Model file for the job. Use its own axes, mm. Face numbers are marked on the shaded views. A direction names the side the tool comes from. Round coordinates to 2 decimals unless told otherwise and drop trailing zeros. Loops run counter-clockwise (first coordinate to the right, second up) from the corner with the lowest first, then second, coordinate; pieces in that order, holes last. Notation, with made-up numbers: M -31.75,65.5 L 8.25,65.5 A21 ccw 8.25,85.5 Z; hole C 6,-9.75 d3. An arc over 180 degrees is marked long. Use a Markdown table: item, result. Add a question column.
Q1. Cut at B-B (x = 114.3). Give the cut face in (y, z), plus the area to 3 significant figures.
Q2. Mould opens along Y. For the marked faces 3, 4 and 5 say: +Y half, -Y half, draft (parallel to the pull), parting line (faces both ways), or undercut.
Q3. Cut at C-C (x = 76.5). Give the cut face in (y, z), plus the area to 3 significant figures.
Q4. Cut at A-A (z = 6.5). Give the cut face in (x, y).
Q5. Tool access for the marked faces 1 and 2: list every direction of +Z, -Z, +X, -X, +Y, -Y with a clear straight run to the whole face (end or side of a thin tool).
Q6. Cut at D-D (x = 57.5). Give the cut face in (y, z), plus the area to 3 significant figures.
Q7. Probe line 1 (Y direction, x = 60, z = 12.5); line 2 (Y direction, x = 99, z = 11.25); line 3 (Z direction, x = 114, y = 1). List the from-to ranges inside material, lowest first. Write a range as from..to.
Q8. Pin check, flat tips, straight feed: pin 1 (1 mm diameter, centred on x = 85.5, y = 18.5, fed in from +Z); pin 2 (7 mm diameter, centred on y = 92.5, z = 16, fed in from +X); pin 3 (2 mm diameter, centred on x = 69.5, z = 12, fed in from -Y); pin 4 (3 mm diameter, centred on x = 49.5, y = 143, fed in from +Z). Stop position of each tip, or through.
from build123d import *

# Parameters (mm, degrees)
SKETCH1_W           = 127
SKETCH1_H           = 147.574
BOSS_EXTRUDE1_DEPTH = 3.81
SKETCH3_W           = 127
SKETCH3_H           = 6.35
BOSS_EXTRUDE2_DEPTH = 16.51
SKETCH4_R           = 3.429
CUT_EXTRUDE1_DEPTH  = 196.754917885
SKETCH6_W           = 12.7
SKETCH6_H           = 6.35
BOSS_EXTRUDE3_DEPTH = 18.796
CUT_EXTRUDE4_DEPTH  = 6.35


with BuildPart() as part:
    # Sketch1 → Boss-Extrude1 (new body)
    with BuildSketch(Plane.XY):
        with Locations((63.5, 73.787)):
            Rectangle(SKETCH1_W, SKETCH1_H)
    extrude(amount=BOSS_EXTRUDE1_DEPTH)

    # Sketch3 → Boss-Extrude2 (add)
    with BuildSketch(Plane.XY.offset(3.81)):
        with Locations((63.5, 144.399)):
            Rectangle(SKETCH3_W, SKETCH3_H)
        with Locations((63.5, 3.175)):
            Rectangle(SKETCH3_W, SKETCH3_H)
    extrude(amount=BOSS_EXTRUDE2_DEPTH)

    # Sketch4 → Cut-Extrude1 (cut, through all)
    with BuildSketch(Plane.XZ):
        with Locations(Location((12.7, 13.462, 0), (0, 0, 270))):
            Circle(SKETCH4_R)
        with Locations(Location((114.3, 13.462, 0), (0, 0, 270))):
            Circle(SKETCH4_R)
    extrude(amount=-CUT_EXTRUDE1_DEPTH, mode=Mode.SUBTRACT)

    # Sketch6 → Boss-Extrude3 (add)
    with BuildSketch(Plane.XY.offset(3.81)):
        with Locations((6.35, 91.694)):
            Rectangle(SKETCH6_W, SKETCH6_H)
        with Locations((59.69, 91.694)):
            Rectangle(SKETCH6_W, SKETCH6_H)
    extrude(amount=BOSS_EXTRUDE3_DEPTH)

    # Sketch10 → Cut-Extrude4 (cut)
    with BuildSketch(Plane.XZ.offset(-88.519)):
        with BuildLine():
            ThreePointArc((59.2, 17.66), (59.397338077, 18.539315257), (59.2169552, 19.422264664))
            ThreePointArc((59.2169552, 19.422264664), (59.208568363, 19.441173113), (59.2, 19.46))
            ThreePointArc((59.2, 19.46), (55.097437581, 18.56), (59.2, 17.66))
        make_face()
    extrude(amount=-CUT_EXTRUDE4_DEPTH, mode=Mode.SUBTRACT)


solid = part.part
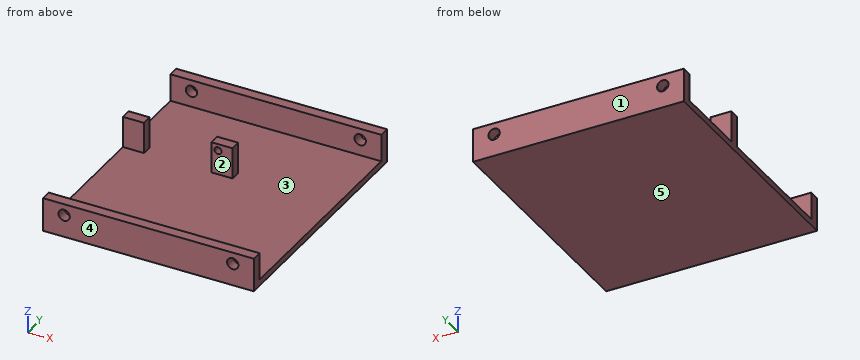
Checked values:
| question | item | result |
|---|---|---|
| 1 | outline | M 0,0 L 147.57,0 L 147.57,10.03 L 141.22,10.03 L 141.22,3.81 L 6.35,3.81 L 6.35,10.03 L 0,10.03 Z; M 0,16.89 L 6.35,16.89 L 6.35,20.32 L 0,20.32 Z; M 141.22,16.89 L 147.57,16.89 L 147.57,20.32 L 141.22,20.32 Z |
| 1 | area | 685 mm^2 |
| 2 | face 3 | undercut |
| 2 | face 4 | -Y half |
| 2 | face 5 | draft |
| 3 | outline | M 0,0 L 147.57,0 L 147.57,20.32 L 141.22,20.32 L 141.22,3.81 L 6.35,3.81 L 6.35,20.32 L 0,20.32 Z |
| 3 | area | 772 mm^2 |
| 4 | outline | M 0,0 L 127,0 L 127,6.35 L 0,6.35 Z; M 0,88.52 L 12.7,88.52 L 12.7,94.87 L 0,94.87 Z; M 0,141.22 L 127,141.22 L 127,147.57 L 0,147.57 Z; M 53.34,88.52 L 66.04,88.52 L 66.04,94.87 L 53.34,94.87 Z |
| 5 | face 1 | +Z, -Z, +X, -X, +Y |
| 5 | face 2 | +Z, +X, -X |
| 6 | outline | M 0,0 L 147.57,0 L 147.57,20.32 L 141.22,20.32 L 141.22,3.81 L 94.87,3.81 L 94.87,16.42 L 88.52,16.42 L 88.52,3.81 L 6.35,3.81 L 6.35,20.32 L 0,20.32 Z; M 88.52,20.7 L 94.87,20.7 L 94.87,22.61 L 88.52,22.61 Z |
| 6 | area | 864 mm^2 |
| 7 | line 1 | y = 0..6.35, 88.52..94.87, 141.22..147.57 |
| 7 | line 2 | y = 0..6.35, 141.22..147.57 |
| 7 | line 3 | z = 0..10.05, 16.88..20.32 |
| 8 | pin 1 | stops at z = 3.81 |
| 8 | pin 2 | stops at x = 66.04 |
| 8 | pin 3 | stops at y = 0 |
| 8 | pin 4 | stops at z = 20.32 |
